```python
from build123d import *

# Parameters (mm, degrees)
F1_DEPTH = 50
F3_DEPTH = 25
F4_DEPTH = 25
F5_W     = 50
F5_H     = 50
F6_DEPTH = 25


with BuildPart() as f1:
    # F0 (on Front) → F1 (new body)
    with BuildSketch(Plane.XZ):
        Polygon((874.097177, 74.70942), (874.097177, 24.70942), (1524.597177, 24.70942), (1574.597177, 74.70942), align=None)
    extrude(amount=F1_DEPTH)

    # F2 (on face) → F3 (cut)
    with BuildSketch(Plane.XZ.offset(50)):
        Polygon((1524.597177, 24.70942), (1574.597177, 74.70942), (1503.886499, 74.70942), (1453.886499, 24.70942), align=None)
    extrude(amount=-F3_DEPTH, mode=Mode.SUBTRACT)

    # F2 (on face) → F4 (cut)
    with BuildSketch(Plane.XZ.offset(50)):
        Polygon((1524.597177, 24.70942), (1574.597177, 74.70942), (1503.886499, 74.70942), (1453.886499, 24.70942), align=None)
    extrude(amount=-F4_DEPTH, mode=Mode.SUBTRACT)

    # F5 (on face) → F6 (cut)
    with BuildSketch(Plane.XZ.offset(50)):
        with Locations((899.097177, 49.70942)):
            Rectangle(F5_W, F5_H)
    extrude(amount=-F6_DEPTH, mode=Mode.SUBTRACT)


solid = f1.part
```
Model file for the job. Use its own axes, mm. A direction names the side the tool comes from. Coordinates: 2 decimals unless noted, no trailing zeros. Loops run counter-clockwise (first coordinate to the right, second up) from the corner with the lowest first, then second, coordinate; pieces in that order, holes last. Notation, with made-up numbers: (23.25, 9) -> (65.25, 9) arc R13 ccw to (65.25, 16) -> close; hole circle Ø3 at (22.5, 47). An arc over 180 degrees is marked (long way). Answer as a JSON object with one key per item and string values.
Q1. Cut at C-C (z = 35). List the corners of the cut face in (x, y).
Report:
{"outline": "(874.1, -25) -> (924.1, -25) -> (924.1, -50) -> (1464.18, -50) -> (1464.18, -25) -> (1534.89, -25) -> (1534.89, 0) -> (874.1, 0) -> close"}
Q2. Cut at B-B (y = -42.5). List the corners of the cut face in (x, z), and give its area (3 significant figures).
Report:
{"outline": "(924.1, 24.71) -> (1453.89, 24.71) -> (1503.89, 74.71) -> (924.1, 74.71) -> close", "area": "27,700 mm2"}
Q3. Cut at D-D (y = -12). List the corners of the cut face in (x, z).
Report:
{"outline": "(874.1, 24.71) -> (1524.6, 24.71) -> (1574.6, 74.71) -> (874.1, 74.71) -> close"}
Q4. Cut at A-A (z = 64). List the corners of the cut face in (x, y), and give its area (3 significant figures).
Report:
{"outline": "(874.1, -25) -> (924.1, -25) -> (924.1, -50) -> (1493.18, -50) -> (1493.18, -25) -> (1563.89, -25) -> (1563.89, 0) -> (874.1, 0) -> close", "area": "31,500 mm2"}
Q5. Probe probe 1 along Y at (x, z) = (1473, 38); probe 2 along X at (y, z) = (-31.5, 36.5); probe 3 along X at (y, z) = (-9, 43.5). List the from-to ranges inside material, lowest first.
Report:
{"probe 1": "y = -25 to 0", "probe 2": "x = 924.1 to 1465.68", "probe 3": "x = 874.1 to 1543.39"}
Q6. 3-axis set-ups, long thin cutter, end or side, ignore diameter. For faces 1 (the flat face through (924.097, -38, 49)), 2 (the flat face through (1549.25, -12.32, 49.36)), 3 (the flat face through (1479.236, -37.675, 50.059)): which of +Z, -Z, +X, -X, +Y, -Y reach the whole face in a straight line?
Report:
{"face 1": "+Z, -Z, -X, -Y", "face 2": "-Z, +X, +Y, -Y", "face 3": "-Z, +X, -Y"}
Q7. Flat gauge pins, fed straight in: P1, Ø25, axis at x = 1524, z = 56.5, coming from the -Y side; P2, Ø6, axis at y = -38, z = 36.5, coming from the -X side; P3, Ø8, axis at y = -17, z = 36, coming from the +X side. Where does each tip first touch, or does it go through?
Report:
{"P1": "stops at y = -25", "P2": "stops at x = 924.1", "P3": "stops at x = 1539.89"}
